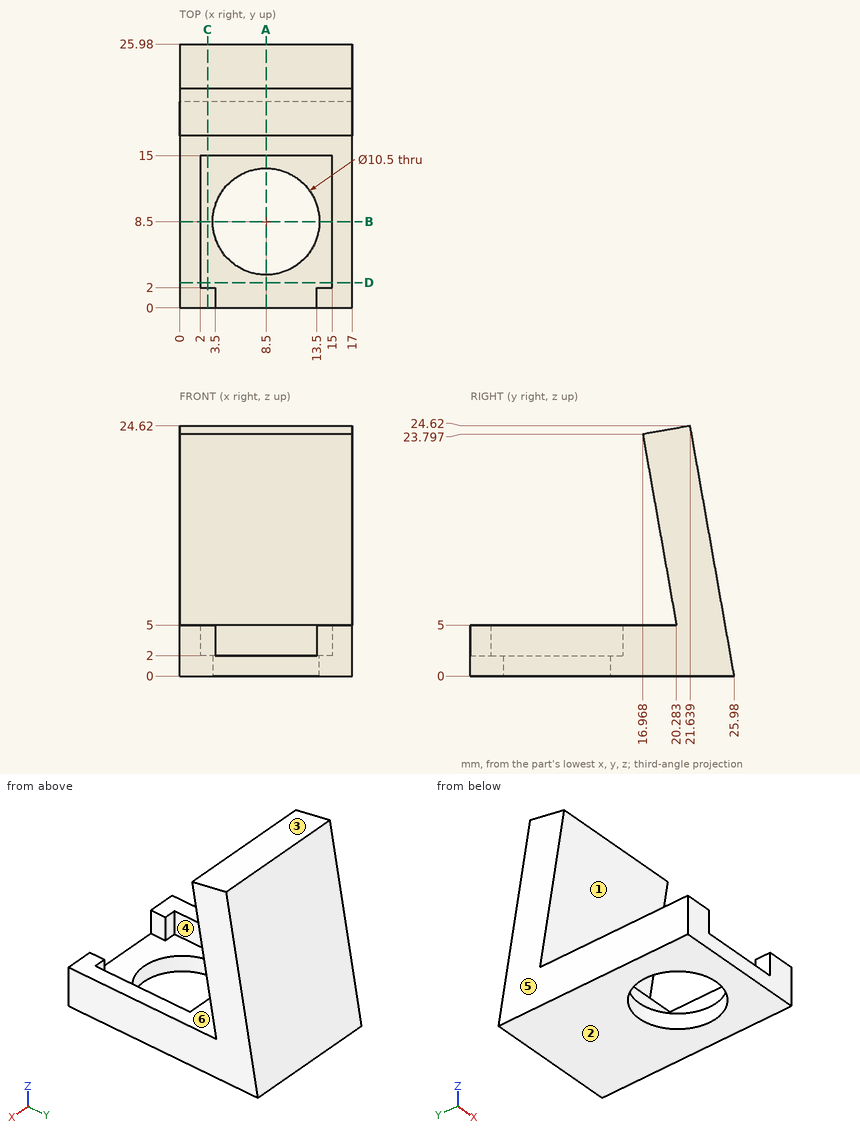
For this review, use the dimensioned drawing (mm, ordinates from the lowest corner) and the shaded views. A direction names the side the tool comes from. Round coordinates to 2 decimals unless told otherwise and drop trailing zeros. Order: outer loops, then holes, each group sorted by start corner. A loop starts at its lowest first (then second) coordinate and runs counter-clockwise, first axis right, second up. Notation, with made-up numbers: M -11,85.25 L 7,85.25 A21 cw 7,90.25 Z; hole C 3.25,85.25 d5. An arc over 180 degrees is marked long. Write each question's results on one line, items separated by ' | '. Start each with the question number.
1. Draft analysis for pull direction Z (two halves, no side actions). For the marked faces 1, 2 and 3, state which applies: pulls with the +Z half, pulls with the -Z half, needs draft (parallel to the pull), parting line crosses it, or undercut.
2. Add section C-C (x = 2.75). State the section outline as (y, z) points.
3. Add section D-D (y = 2.5). State the section outline as (x, z) points, then the cut area to 3 significant figures.
4. Tool access review of the marked faces 4, 5 and 6: name each direction out of +Z, -Z, +X, -X, +Y, -Y from which nothing blocks a thin tool from reaching the whole face with its end or side.
5. To check wall thickness, follow L1, parallel to X at y = 9, z = 3.5; L2, parallel to Z at x = 8, y = 14.5; L3, parallel to Z at x = 1.75, y = 10.25. State the ranges of each line that lie inside material, in increasing order. Write a range as [from, to].
6. Add section A-A (x = 8.5). State the section outline as (y, z) points, then the cut area to 3 significant figures.
7. Add section B-B (y = 8.5). State the section outline as (x, z) points.
8. Clearance check with flat-ended pins moving along their axes: pin 1 Ø8 at (x, y) = (5.5, 5.5) entering from +Z; pin 2 Ø1.6 at (x, z) = (2.5, 4) entering from +Y; pin 3 Ø6 at (x, z) = (3.5, 16) entering from -Y. State where each tip first meets the part, or that it passes through.
Output values:
1) face 1: undercut | face 2: pulls with the -Z half | face 3: pulls with the +Z half
2) outline: M 0,0 L 25.98,0 L 21.64,24.62 L 16.97,23.8 L 20.28,5 L 15,5 L 15,2 L 2,2 L 2,5 L 0,5 Z
3) outline: M 0,0 L 17,0 L 17,5 L 15,5 L 15,2 L 2,2 L 2,5 L 0,5 Z | area: 46.0 mm^2
4) face 4: +Z | face 5: +Z, -Z, -X, +Y, -Y | face 6: +X, -X, -Y
5) L1: [0, 2], [15, 17] | L2: [0, 2] | L3: [0, 5]
6) outline: M 0,0 L 3.25,0 L 3.25,2 L 0,2 Z; M 13.75,0 L 25.98,0 L 21.64,24.62 L 16.97,23.8 L 20.28,5 L 15,5 L 15,2 L 13.75,2 Z | area: 154 mm^2
7) outline: M 0,0 L 3.25,0 L 3.25,2 L 2,2 L 2,5 L 0,5 Z; M 13.75,0 L 17,0 L 17,5 L 15,5 L 15,2 L 13.75,2 Z
8) pin 1: z = 5 | pin 2: y = 25.42 | pin 3: y = 17.81
